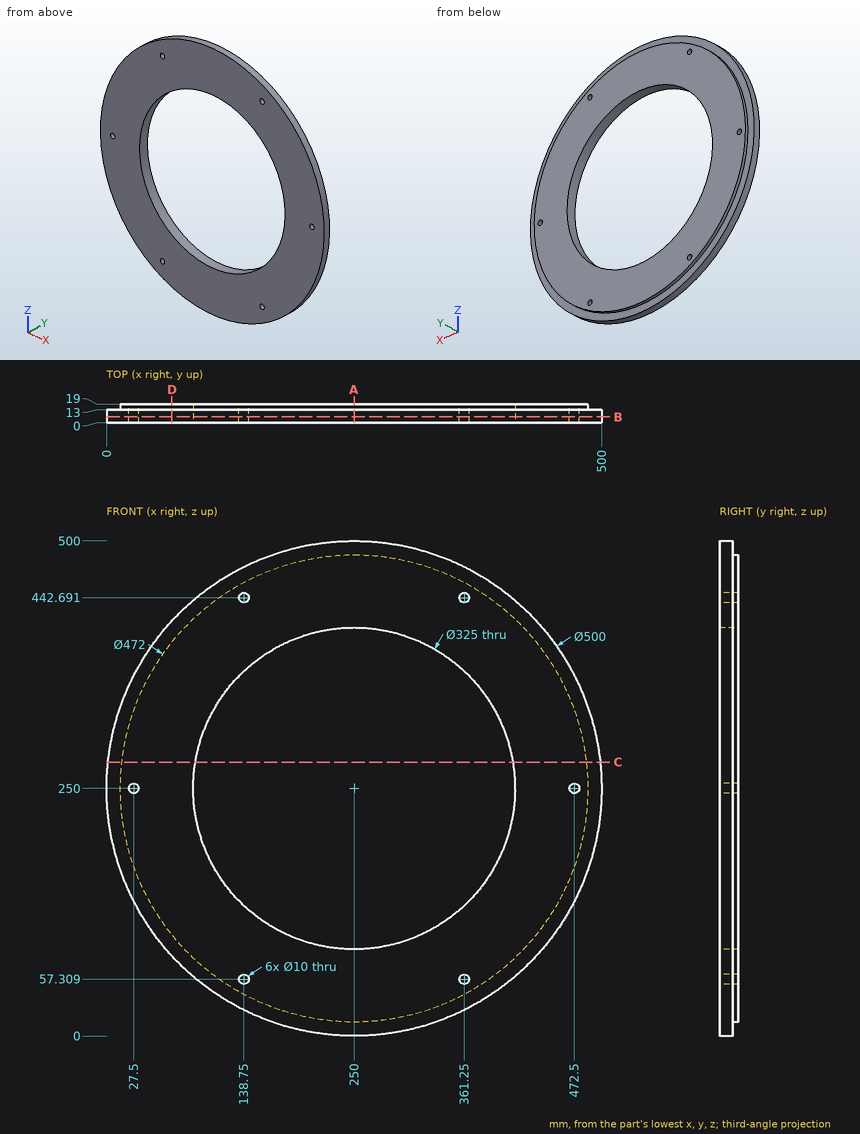
Could you check a few things on this drawing? It's one solid part, dimensions in mm from its lowest x, y, z. Round coordinates to 2 decimals unless told otherwise and drop trailing zeros. Write each loop counter-clockwise with the first axis right and the second up, starting at its lowest first coordinate (ties: lowest second). Pieces come first, ordered by that corner, then holes.
Q1. If we section it at D-D on x = 66: Write out the boundary of the cut face in (y, z) (1 decimal).
Q2. If we section it at B-B on y = 6: Write out the boundary of the cut face in (x, z), plus the area to 3 significant figures.
Q3. If we section it at A-A on x = 250: Write out the boundary of the cut face in (y, z), plus the area to 3 significant figures.
Q4. Will these pins go through, and if not, where does the flat tip stop? P1, Ø4, axis at x = 155.5, y = 7, coming from the +Z side; P2, Ø8, axis at x = 300, y = 2.5, coming from the +Z side; P3, Ø8, axis at x = 361.25, z = 442.69, coming from the +Y side; P4, Ø1.5, axis at y = 16.5, z = 145, coming from the -X side.
Q5. Please list where these lines run through material, in increasing order: probe 1 along X at (y, z) = (15.25, 250); probe 2 along X at (y, z) = (6.75, 250); probe 3 along Z at (x, y) = (361.25, 6.5) (1 decimal).
Q6. If we section it at C-C on z = 276.5: Write out the boundary of the cut face in (x, y) (1 decimal).
Answer below:
1. outline: (0, 80.8) - (13, 80.8) - (13, 102.2) - (19, 102.2) - (19, 397.8) - (13, 397.8) - (13, 419.2) - (0, 419.2) - close
2. outline: circle Ø500 at (250, 250); hole circle Ø10 at (27.5, 250); hole circle Ø325 at (250, 250); hole circle Ø10 at (138.75, 57.31); hole circle Ø10 at (138.75, 442.69); hole circle Ø10 at (361.25, 57.31); hole circle Ø10 at (361.25, 442.69); hole circle Ø10 at (472.5, 250)
2. area: 113,000 mm2
3. outline: (0, 0) - (13, 0) - (13, 14) - (19, 14) - (19, 87.5) - (0, 87.5) - close; (0, 412.5) - (19, 412.5) - (19, 486) - (13, 486) - (13, 500) - (0, 500) - close
3. area: 3,160 mm2
4. P1: stops at z = 482.26
4. P2: stops at z = 495.73
4. P3: passes through
4. P4: stops at x = 38.27
5. probe 1: x = 14 to 22.5, 32.5 to 87.5, 412.5 to 467.5, 477.5 to 486
5. probe 2: x = 0 to 22.5, 32.5 to 87.5, 412.5 to 467.5, 477.5 to 500
5. probe 3: z = 26.1 to 52.3, 62.3 to 131.6, 368.4 to 437.7, 447.7 to 473.9
6. outline: (1.4, 0) - (89.7, 0) - (89.7, 19) - (15.5, 19) - (15.5, 13) - (1.4, 13) - close; (410.3, 0) - (498.6, 0) - (498.6, 13) - (484.5, 13) - (484.5, 19) - (410.3, 19) - close
